Here's how the part is built. I have some questions about the finished solid (model axes, mm). A direction names the side the tool comes from. Round coordinates to 2 decimals unless told otherwise and drop trailing zeros. Loops run counter-clockwise (first coordinate to the right, second up) from the corner with the lowest first, then second, coordinate; pieces in that order, holes last. Notation, with made-up numbers: M -19.5,60.25 L -5.5,60.25 A22 ccw -5.5,87.25 Z; hole C -19.75,46 d7. An arc over 180 degrees is marked long. Answer as CSV lines item,"result".
Autodesk Inventor part; units mm, degrees
ref_plane "YZ Plane" through (0, 0, 0) normal (1, 0, 0) x (0, 1, 0)
ref_plane "XZ Plane" through (0, 0, 0) normal (0, 1, 0) x (-1, 0, 0)
ref_plane "XY Plane" through (0, 0, 0) normal (0, 0, 1) x (1, 0, 0)
sketch "Sketch5" plane through (0, 0, 0) normal (0, 0, 1) x (1, 0, 0)
  line L0 (52.8, -15.6) -> (52.8, -10.6)
  line L1 (52.8, -10.6) -> (49.8, -10.6)
  line L2 (49.8, -10.6) -> (49.8, -12.55)
  line L3 (44, -12.55) -> (44, -3.05)
  line L4 (49.8, -3.05) -> (49.8, -5)
  line L5 (49.8, -5) -> (52.8, -5)
  line L6 (52.8, -5) -> (52.8, 0)
  line L7 (52.8, 0) -> (7.8, 0)
  line L8 (44, -3.05) -> (49.8, -3.05)
  line L9 (44, -12.55) -> (49.8, -12.55)
  line L10 (52.8, -15.6) -> (7.8, -15.6)
  arc A0 (7.8, 0) -> (7.8, -15.6) centre (7.8, -7.8) ccw
  point P0 (0, 0)
  dimension "d41" = 5.8
  dimension "d48" = 44
  dimension "d50" = 3
  dimension "d63" = 45
  dimension "d67" = 15.6
  dimension "d71" = 0
  dimension "d72" = 36.2
  dimension "d80" = 5.6
  dimension "d81" = 9.5
extrude "Extrusion2" add sketch "Sketch5" along normal blind 12
sketch "Sketch7" plane through (0, 0, 12) normal (0, 0, 1) x (1, 0, 0)
  line L0 (52.8, 0) -> (7.8, 0)
  line L1 (7.8, 0) -> (0, 0)
  line L2 (0, 0) -> (0, -15.6)
  line L3 (0, -15.6) -> (7.8, -15.6)
  line L4 (7.8, -15.6) -> (7.8, 0)
  point P0 (0, 0)
extrude "Extrusion4" cut sketch "Sketch7" against normal through all
sketch "Sketch9" plane through (0, 0, 12) normal (0, 0, 1) x (1, 0, 0)
  line L0 (52.8, 0) -> (7.8, 0)
  line L1 (7.8, 0) -> (-6.9721, -2.6047)
  line L2 (-6.9721, -2.6047) -> (-4.2632, -17.9677)
  line L3 (-4.2632, -17.9677) -> (10.5089, -15.363)
  line L4 (7.8, 0) -> (10.5089, -15.363)
  line L5 (7.8, 0) -> (7.8, -15.6)
  point P0 (0, 0)
  dimension "d83" = 15.6
  dimension "d84" = 10
  dimension "d85" = 90
  dimension "d86" = 10
  dimension "d87" = 15
extrude "Extrusion5" add sketch "Sketch9" against normal up to surface (12 mm away)
equation "\"l1\" = 8"
properties part number "Finray_test_8_Flach_winkel10deg"
1. I want a section at A-A, the plane y = -11.25. Please give me the cut outline in (x, z).
Evaluation:
outline,"M -5.45,0 L 44,0 L 44,12 L -5.45,12 Z; M 49.8,0 L 52.8,0 L 52.8,12 L 49.8,12 Z"
2. Which directions (+Z, -Z, +X, -X, +Y, -Y) give clear straight access to the entire face, cutting with the end or side of a thin tool? Please do faces 4 (the flat face through (31, -15.6, 6)), 5 (the flat face through (51, -5, 6)), 6 (the flat face through (49.8, -4, 6)).
Evaluation:
face 4,"+Z, -Z, +X, -Y"
face 5,"+Z, -Z, +X"
face 6,"+Z, -Z"
3. If I drill on line 1 (Y direction, x = 44.5, z = 7.25); line 2 (Y direction, x = 29, z = 1.25); line 3 (X direction, y = -12, z = 2.75), over which ranges is the centre line in solid material (lowest first)? Write a range as [from, to].
Evaluation:
line 1,"y = [-15.6, -12.55], [-3.05, 0]"
line 2,"y = [-15.6, 0]"
line 3,"x = [-5.32, 44], [49.8, 52.8]"
4. I want a section at D-D, the plane y = -9. Please give me the cut outline in (x, z), and give its area (3 significant figures).
Evaluation:
outline,"M -5.84,0 L 44,0 L 44,12 L -5.84,12 Z"
area,"598 mm²"
5. I want a section at B-B, the plane z = 11. Please give me the cut outline in (x, y), and give its area (3 significant figures).
Evaluation:
outline,"M -6.97,-2.6 L -4.26,-17.97 L 9.16,-15.6 L 52.8,-15.6 L 52.8,-10.6 L 49.8,-10.6 L 49.8,-12.55 L 44,-12.55 L 44,-3.05 L 49.8,-3.05 L 49.8,-5 L 52.8,-5 L 52.8,0 L 7.8,0 Z"
area,"843 mm²"
6. We'd pull the mould along X, two halves only. Please class faces 1 (the flat face through (31, 0, 6)), 2 (the flat face through (49.8, -12, 6)), 3 (the flat face through (2.36, -16.8, 6.08)): pulls with the +X half, pulls with the -X half, needs draft (parallel to the pull), parting line crosses it, or undercut.
Evaluation:
face 1,"needs draft"
face 2,"undercut"
face 3,"pulls with the +X half"
7. I want a section at C-C, the plane x = 14.5. Please give me the cut outline in (y, z), and give its area (3 significant figures).
Evaluation:
outline,"M -15.6,0 L 0,0 L 0,12 L -15.6,12 Z"
area,"187 mm²"
8. For P1, Ø1.5, axis at y = -5.5, z = 10, coming from the -X side; P2, Ø4, axis at x = 42.5, z = 7.5, coming from the -Y side; P3, Ø2, axis at y = -4, z = 6, coming from the -X side, each with a flat end and sliding along its axis, tell me the tip position at first contact or that it passes through.
Evaluation:
P1,"stops at x = -6.59"
P2,"stops at y = -15.6"
P3,"stops at x = -6.9"
